Work out the finished part from the listing and answer in its coordinate system (mm). A direction names the side the tool comes from. Coordinates: 2 decimals unless noted, no trailing zeros. Loops run counter-clockwise (first coordinate to the right, second up) from the corner with the lowest first, then second, coordinate; pieces in that order, holes last. Notation, with made-up numbers: (28.5, 13) -> (47.5, 13) arc R26 cw to (47.5, 44) -> close; hole circle Ø1 at (79.25, 58.5). An arc over 180 degrees is marked (long way). Use a Markdown table: item, result.
Autodesk Inventor part; units mm, degrees
ref_plane "YZ Plane" through (0, 0, 0) normal (1, 0, 0) x (0, 1, 0)
ref_plane "XZ Plane" through (0, 0, 0) normal (0, 1, 0) x (-1, 0, 0)
ref_plane "XY Plane" through (0, 0, 0) normal (0, 0, 1) x (1, 0, 0)
sketch "Sketch1" plane through (0, 0, 0) normal (0, 1, 0) x (-1, 0, 0)
  line L0 (0, 0) -> (0, -18.7068)
  line L1 (0, -18.7068) -> (19.6073, -91.8823)
  line L2 (0, 0) -> (0, 11.24)
  line L3 (0, 11.24) -> (14, 11.24)
  line L4 (14, 11.24) -> (14, -13)
  line L5 (14, -13) -> (34.0962, -88)
  line L6 (34.0962, -88) -> (19.6073, -91.8823)
  dimension "d1" = 14
  dimension "d2" = 11.24
  dimension "d4" = 15
  dimension "d13" = 15
  dimension "d14" = 13
  dimension "d35" = 88
extrude "Extrusion1" add sketch "Sketch1" along normal blind 183
sketch "Sketch2" plane through (-14, 0, -13) normal (-1, 0, 0) x (0, 0, 1)
  line L0 (0, 183) -> (24.24, 183)
  circle A0 centre (12.74, 171.5) radius 4.25
  circle A1 centre (12.74, 11.5) radius 4.25
  line L1 (24.24, 0) -> (24.24, 183)
  line L2 (0, 0) -> (24.24, 0)
  arc A2 (12.74, 0) -> (15.1193, 22.7512) centre (12.74, 11.5) ccw
  arc A3 (12.2608, 160.01) -> (12.74, 183) centre (12.74, 171.5) ccw
  line L3 (-13.26, 102.4155) -> (-13.26, 135.5313)
  arc A4 (12.2608, 160.01) -> (-13.26, 135.5313) centre (11.24, 135.5313) ccw
  circle A5 centre (20.1015, 118.5) radius 28 construction
  line L4 (12.74, 25.6863) -> (12.74, 74.0254)
  arc A6 (12.74, 25.6863) -> (15.1193, 22.7512) centre (15.74, 25.6863) ccw
  arc A7 (-13.26, 102.4155) -> (9.0909, 78.01) centre (11.24, 102.4155) ccw
  arc A8 (12.74, 74.0254) -> (9.0909, 78.01) centre (8.74, 74.0254) ccw
  line L5 (24.24, 0) -> (24.24, 183)
  line L6 (12.74, 0) -> (24.24, 0)
  line L7 (24.24, 11.5) -> (24.24, 171.5)
  line L8 (24.24, 183) -> (12.74, 183)
  line L9 (24.24, 11.5) -> (24.24, 0)
  line L10 (24.24, 171.5) -> (24.24, 183)
  point P0 (13, 0)
  point P1 (12.74, 23)
  point P2 (12.74, 77.9615)
  dimension "d17" = 160
  dimension "d18" = 183
  dimension "d19" = 11.5
  dimension "d20" = 11.5
  dimension "d21" = 11.5
  dimension "d22" = 26
  dimension "d23" = 56
  dimension "d24" = 53
  dimension "d25" = 3
  dimension "d26" = 0
  dimension "d27" = 24.5
  dimension "d28" = 4
  dimension "d30" = 82
  dimension "d31" = 8.5
  dimension "d32" = 4.1385
extrude "Extrusion2" cut sketch "Sketch2" along normal through all both and the other way through all
sketch "Sketch3" plane through (-34.0962, 0, -88) normal (-0.9659258, 0, 0.258819) x (0.258819, 0, 0.9659258)
  line L0 (46.9516, 11.5) -> (72.9516, 11.5)
  line L1 (72.9516, 11.5) -> (72.9516, 56.75)
  line L2 (72.9516, 56.75) -> (46.9516, 56.75)
  line L3 (46.9516, 56.75) -> (46.9516, 11.5)
  ellipse E0 centre (89.9516, 11.5) end of major axis (89.9516, 23) minor radius 11.1081 (89.9516, 0) -> (92.2498, 22.7512) ccw
  line L4 (8.9516, 106.5) -> (34.9516, 106.5)
  line L5 (34.9516, 106.5) -> (34.9516, 174.5)
  line L6 (34.9516, 174.5) -> (8.9516, 174.5)
  line L7 (8.9516, 174.5) -> (8.9516, 106.5)
  circle A0 centre (6.4516, 103) radius 1.4
  circle A1 centre (37.4516, 103) radius 1.4
  circle A2 centre (37.4516, 178) radius 1.4
  circle A3 centre (6.4516, 178) radius 1.4
  line L8 (6.4516, 103) -> (37.4516, 103) construction
  line L9 (37.4516, 103) -> (37.4516, 178) construction
  line L10 (37.4516, 178) -> (6.4516, 178) construction
  line L11 (6.4516, 178) -> (6.4516, 103) construction
  point P0 (93.8262, 0)
  dimension "d36" = 45.25
  dimension "d37" = 26
  dimension "d38" = 17
  dimension "d39" = 0
  dimension "d46" = 26
  dimension "d47" = 31
  dimension "d48" = 75
  dimension "d49" = 3.5
  dimension "d50" = 68
  dimension "d51" = 2.5
  dimension "d52" = 55
  dimension "d53" = 95
  dimension "d54" = 2.8
extrude "top" cut sketch "Sketch3" against normal blind 183
sketch "Sketch4" plane through (-19.6073, 0, -91.8823) normal (0.9659258, 0, -0.258819) x (-0.258819, 0, -0.9659258)
  line L0 (-46.9516, 56.75) -> (-46.9516, 11.5)
  line L1 (-72.9516, 11.5) -> (-72.9516, 56.75)
  line L2 (-42.9516, 56.75) -> (-76.9516, 56.75)
  line L3 (-76.9516, 56.75) -> (-76.9516, 11.5)
  line L4 (-76.9516, 11.5) -> (-42.9516, 11.5)
  line L5 (-42.9516, 11.5) -> (-42.9516, 56.75)
  line L6 (-72.9516, 56.75) -> (-46.9516, 56.75)
  line L7 (-46.9516, 11.5) -> (-72.9516, 11.5)
  line L8 (-3.9516, 180.5) -> (-39.9516, 180.5)
  line L9 (-39.9516, 180.5) -> (-39.9516, 100.5)
  line L10 (-39.9516, 100.5) -> (-3.9516, 100.5)
  line L11 (-3.9516, 100.5) -> (-3.9516, 180.5)
  circle A0 centre (-6.4516, 103) radius 1.4
  circle A1 centre (-6.4516, 178) radius 1.4
  circle A2 centre (-37.4516, 178) radius 1.4
  point P0 (-93.8262, 0)
  dimension "d42" = 4
  dimension "d43" = 4
  dimension "d55" = 2.5
  dimension "d56" = 2.5
  dimension "d57" = 2.5
  dimension "d59" = 2.5
extrude "back" cut sketch "Sketch4" against normal blind 12.6 contours L2 L5 L4 L0 | L1 L4 L3 L2 | L11 L10 L9 L8
equation "\"d19\" = -0.5 * d17 + 0.5 * d18"
equation "\"d21\" = d20"
equation "\"d49\" = -0.5 * d50 + 0.5 * d48"
equation "\"d51\" = -0.5 * d46 + 0.5 * d47"
equation "\"d43\" = d42"
equation "\"d56\" = d55"
equation "\"d57\" = d55"
equation "\"d59\" = d55"
properties part number "dash"
Q1. Consider line 1 (Y direction, x = -24, z = -58.5); line 2 (Y direction, x = -20.5, z = -78); line 3 (Y direction, x = -8, z = -3.5). Determine where each line is inside the solid, lowest interval first. Write a range as [from, to].
Solved:
| item | result |
|---|---|
| line 1 | [0, 106.5], [174.5, 183] |
| line 2 | [0, 100.5], [180.5, 183] |
| line 3 | [0, 8.75], [14.25, 77.95], [159.97, 168.75], [174.25, 183] |
Q2. Section D-D on y = 65.5 is taken. Determine the outline of the cut face in (x, z), and give its area (3 significant figures).
Solved:
| item | result |
|---|---|
| outline | (-34.1, -88) -> (-19.61, -91.88) -> (0, -18.71) -> (0, -0.26) -> (-14, -0.26) -> (-14, -13) -> close |
| area | 1,370 mm² |
Q3. Section A-A on y = 110 is taken. Determine the outline of the cut face in (x, z), and give its area (3 significant figures).
Solved:
| item | result |
|---|---|
| outline | (-34.1, -88) -> (-19.61, -91.88) -> (-18.58, -88.07) -> (-30.76, -84.8) -> (-29.46, -79.97) -> (-31.78, -79.35) -> close; (-25.05, -54.24) -> (-22.73, -54.86) -> (-21.44, -50.03) -> (-9.27, -53.29) -> (-2.02, -26.26) -> (-17.55, -26.26) -> close |
| area | 473 mm² |
Q4. Section C-C on z = -8.5 is taken. Determine the outline of the cut face in (x, y), and give its area (3 significant figures).
Solved:
| item | result |
|---|---|
| outline | (-14, 0) -> (0, 0) -> (0, 78.86) -> (-14, 78.86) -> close; (-14, 159.09) -> (0, 159.09) -> (0, 183) -> (-14, 183) -> close |
| area | 1,440 mm² |
Q5. Section B-B on y = 171.5 is taken. Determine the outline of the cut face in (x, z), and give its area (3 significant figures).
Solved:
| item | result |
|---|---|
| outline | (-34.1, -88) -> (-19.61, -91.88) -> (-18.58, -88.07) -> (-30.76, -84.8) -> (-29.46, -79.97) -> (-31.78, -79.35) -> close; (-25.05, -54.24) -> (-22.73, -54.86) -> (-21.44, -50.03) -> (-9.27, -53.29) -> (0, -18.71) -> (0, -4.51) -> (-14, -4.51) -> (-14, -13) -> close; (-14, 3.99) -> (0, 3.99) -> (0, 11.24) -> (-14, 11.24) -> close |
| area | 895 mm² |
Q6. Given pin 1 Ø6 at (x, y) = (-24.5, 18.5) entering from +Z; pin 2 Ø10 at (x, z) = (-15, -30.5) entering from -Y; pin 3 Ø15.5 at (x, y) = (-8.5, 40) entering from +Z; pin 4 Ø19.5 at (y, z) = (27.5, -2) entering from -X, each flat-ended and moving along its own axis, determine where each tip first touches the part or whether it passes through.
Solved:
| item | result |
|---|---|
| pin 1 | z = -42.65 |
| pin 2 | y = 0 |
| pin 3 | z = -0.26 |
| pin 4 | x = -14 |
Q7. Determine the mould class of faces 1 (the flat face through (-14, 167, -1)), 2 (the flat face through (-15.268, 141.06, -51.684)), 3 (the cylindrical face through (-6.9, 171.52, 11.24)) for opening direction X: pulls with the +X half, pulls with the -X half, needs draft (parallel to the pull), parting line crosses it, or undercut.
Solved:
| item | result |
|---|---|
| face 1 | pulls with the -X half |
| face 2 | undercut |
| face 3 | needs draft |
Q8. For faces 4 (the cylindrical face through (-7.098, 175.714, -0.813)), 5 (the flat face through (-12.374, 34.442, -16.196)), 6 (the flat face through (-27, 90.2, -89.9)), 7 (the flat face through (-7, 50, -0.26)), 8 (the flat face through (-24.586, 139.94, -86.457)), determine the directions among +Z, -Z, +X, -X, +Y, -Y from which every point of the face is accessible in a straight line to the end or side of a thin tool.
Solved:
| item | result |
|---|---|
| face 4 | +X, -X |
| face 5 | none |
| face 6 | -Z, -X, +Y, -Y |
| face 7 | +Z, +X, -X |
| face 8 | +X |
